Design review of the part built by this model. Coordinates are the model's own, in mm. A direction names the side the tool comes from. Coordinates: 2 decimals unless noted, no trailing zeros. Loops run counter-clockwise (first coordinate to the right, second up) from the corner with the lowest first, then second, coordinate; pieces in that order, holes last. Notation, with made-up numbers: M 18.25,0 L 46.25,0 A31 cw 46.25,26 Z; hole C 63.25,-31 d11. An arc over 180 degrees is marked long. Answer as a JSON object with one key per item and string values. Group by question number.
1. Insertion check: pin 1 (5 mm diameter, centred on x = 16, z = 11, fed in from +Y); pin 2 (2 mm diameter, centred on x = -34.5, z = -5.5, fed in from +Y); pin 3 (1.8 mm diameter, centred on y = 2.5, z = -10.5, fed in from -X); pin 4 (1.9 mm diameter, centred on x = -39.85, z = -29.5, fed in from +Y). Each pin has a flat end and moves straight along its axis. Give the tip position at first contact, or say it passes through.
2. Draft analysis for pull direction X (two halves, no side actions). For faces 1 (the cylindrical face through (29.294, 1.59, -30.383)), 2 (the flat face through (-6, -2, 0)), 3 (the flat face through (12, 4, 22)), 4 (the flat face through (32.54, 2, 0)), state which applies: +X half, -X half, draft (parallel to the pull), parting line (faces both ways), or undercut.
3. Consider section D-D (y = 2.5). State the section outline as (x, z) points.
4. To check wall thickness, follow probe 1 along Z at (x, y) = (14, 2.25); probe 2 along X at (y, z) = (3.25, 0.5); probe 3 along X at (y, z) = (-1, 18). State the ranges of each line that lie inside material, in increasing order.
5. Consider section C-C (x = 20). State the section outline as (y, z) points.
6. Machinability: for faces 5 (the flat face through (-1, 2, 23.04)), 6 (the flat face through (-24.65, -1, 0)), 7 (the flat face through (-6, 5.08, -30)), 8 (the flat face through (-6, 2, -31.748)), 9 (the flat face through (-1, 2, 20.5)), which of the approach directions +Z, -Z, +X, -X, +Y, -Y give a long, thin tool a straight path to every point of the face, cutting with its end or side? Answer none if there is none.
7. Consider section A-A (x = -39.85). State the section outline as (y, z) points.
8. Consider section B-B (z = 17). State the section outline as (x, y) points, then the cut area to 3 significant figures.
Autodesk Inventor part; units mm, degrees
ref_plane "YZ Plane" through (0, 0, 0) normal (1, 0, 0) x (0, 1, 0)
ref_plane "XZ Plane" through (0, 0, 0) normal (0, 1, 0) x (-1, 0, 0)
ref_plane "XY Plane" through (0, 0, 0) normal (0, 0, 1) x (1, 0, 0)
sketch "Sketch1" plane through (0, 0, 0) normal (0, 1, 0) x (-1, 0, 0)
  line L0 (31, 20.5) -> (-30, 20.5)
  line L1 (-30, 20.5) -> (-30, -20.5)
  line L2 (-30, -20.5) -> (31, -20.5)
  line L3 (31, -20.5) -> (31, 20.5)
  line L4 (33.54, 23.04) -> (-32.54, 23.04)
  line L5 (-32.54, 23.04) -> (-32.54, -23.04)
  line L6 (-32.54, -23.04) -> (33.54, -23.04)
  line L7 (33.54, -23.04) -> (33.54, 23.04)
  line L8 (-12, -20.5) -> (-12, 20.5)
  line L9 (-12, -23.04) -> (-12, -20.5)
  line L10 (-12, 20.5) -> (-12, 23.04)
  point P0 (0, 0)
  dimension "d0" = 41
  dimension "d1" = 61
  dimension "d2" = 20.5
  dimension "d3" = 31
  dimension "d4" = 2.54
  dimension "d9" = 18
  dimension "d48" = 46.08
extrude "Extrusion1" add sketch "Sketch1" along normal blind 3.5 contours L0 L10 L4 L7 L6 L9 L2 L3
extrude "Extrusion3" add sketch "Sketch1" along normal blind 5.08 contours L0 L1 L2 L9 L6 L5 L4 L10
sketch "Sketch3" plane through (0, 0, 0) normal (0, -1, 0) x (1, 0, 0)
  line L0 (-31, -20.5) -> (30, -20.5)
  line L1 (-31, 20.5) -> (-31, -20.5)
  line L2 (30, 20.5) -> (-31, 20.5)
  line L3 (30, -20.5) -> (30, 20.5)
  line L4 (32.54, -23.04) -> (-33.54, -23.04)
  line L5 (32.54, 23.04) -> (32.54, -23.04)
  line L6 (-33.54, 23.04) -> (32.54, 23.04)
  line L7 (-33.54, -23.04) -> (-33.54, 23.04)
  point P0 (0, 0)
extrude "Extrusion4" add sketch "Sketch3" along normal blind 1 contours L1 L2 L3 L0 | L4 L7 L6 L5
sketch "Sketch4" plane through (0, 0, 0) normal (0, 1, 0) x (1, 0, 0)
  line L0 (12, -20.5) -> (-31, -20.5)
  line L1 (-31, -20.5) -> (-31, 20.5)
  line L2 (30, 20.5) -> (30, -20.5)
  line L3 (30, -20.5) -> (12, -20.5)
  line L4 (-31, 20.5) -> (12, 20.5)
  line L5 (-24.65, 20.5) -> (-20.459, 20.5)
  line L6 (-20.459, 20.5) -> (-20.459, -20.5)
  line L7 (-20.459, -20.5) -> (-24.65, -20.5)
  line L8 (-24.65, -20.5) -> (-24.65, 20.5)
  line L9 (16.03, -20.5) -> (11.839, -20.5)
  line L10 (11.839, -20.5) -> (11.839, 20.5)
  line L11 (11.839, 20.5) -> (16.03, 20.5)
  line L12 (16.03, 20.5) -> (16.03, -20.5)
  point P0 (0, 0)
  point P1 (-24.65, -20.5)
  dimension "d31" = 4.191
  dimension "d37" = 4.191
  dimension "d38" = 13.97
  dimension "d45" = 6.35
extrude "Extrusion5" cut sketch "Sketch4" against normal blind 25.4 contours L0 L10 L4 L11 L12 L3 | L0 L8 L4 L6
sketch "Sketch6" plane through (0, 0, 0) normal (0, 1, 0) x (1, 0, 0)
  line L0 (30, 20.5) -> (-31, 20.5)
  line L1 (30, -20.5) -> (16.03, -20.5)
  line L2 (30, 20.5) -> (27, 20.5)
  line L3 (27, 20.5) -> (27, -20.5)
  line L4 (27, -20.5) -> (30, -20.5)
  line L5 (30, -20.5) -> (30, 20.5)
  point P0 (0, 0)
  dimension "d33" = 3
extrude "Extrusion7" cut sketch "Sketch6" against normal blind 25.4
sketch "Sketch7" plane through (0, 0, 0) normal (0, 1, 0) x (1, 0, 0)
  line L0 (11.839, -20.5) -> (16.03, -20.5)
  line L1 (27, -20.5) -> (27, 20.5)
  line L2 (16.03, -20.5) -> (27, -20.5)
  line L3 (27, -20.5) -> (27, -16.69)
  line L4 (27, -16.69) -> (16.03, -16.69)
  line L5 (16.03, -16.69) -> (16.03, -20.5)
  line L6 (27, -20.5) -> (16.03, -20.5)
  line L7 (19.6495, -16.69) -> (22.1895, -16.69)
  line L8 (22.1895, -20.5) -> (19.6495, -20.5)
  point P0 (0, 0)
  dimension "d39" = 3.81
  dimension "d41" = 10.97
extrude "Extrusion8" cut sketch "Sketch7" against normal blind 25.4
sketch "Sketch9" plane through (0, -1, 0) normal (0, -1, 0) x (1, 0, 0)
  line L0 (32.54, 31.7522) -> (-43.66, 31.7522)
  line L1 (-43.66, 31.7522) -> (-43.66, -31.7478)
  line L2 (-43.66, -31.7478) -> (32.54, -31.7478)
  line L3 (32.54, -31.7478) -> (32.54, 31.7522)
  line L4 (32.54, -23.04) -> (32.54, 23.04)
  line L5 (-33.54, 23.04) -> (-33.54, -23.04)
  line L6 (27, 16.69) -> (16.03, 16.69)
  line L7 (16.03, 16.69) -> (16.03, -20.5)
  line L8 (16.03, -20.5) -> (11.839, -20.5)
  line L9 (11.839, -20.5) -> (11.839, 20.5)
  line L10 (11.839, 20.5) -> (30, 20.5)
  line L11 (30, 20.5) -> (30, -20.5)
  line L12 (30, -20.5) -> (27, -20.5)
  line L13 (27, -20.5) -> (27, 16.69)
  line L14 (-20.459, 20.5) -> (-20.459, -20.5)
  line L15 (-20.459, -20.5) -> (-24.65, -20.5)
  line L16 (-24.65, -20.5) -> (-24.65, 20.5)
  line L17 (-24.65, 20.5) -> (-20.459, 20.5)
  line L18 (32.54, 23.04) -> (-33.54, 23.04)
  line L19 (-33.54, 23.04) -> (-33.54, -23.04)
  line L20 (-33.54, -23.04) -> (32.54, -23.04)
  line L21 (32.54, -23.04) -> (32.54, 23.04)
  point P0 (0, 0)
  point P1 (-33.54, -23.04)
  dimension "d46" = 0
  dimension "d49" = 8.7122
  dimension "d50" = 63.5
  dimension "d51" = 8.7078
  dimension "d52" = 76.2
extrude "Extrusion9" add sketch "Sketch9" against normal blind 1 contours L3 L18 L5 L20 L2 L1 L0
sketch "Sketch10" plane through (0, 0, 0) normal (0, 1, 0) x (1, 0, 0)
  circle A0 centre (-39.85, 29.4978) radius 1.05
  line L0 (-43.66, 31.7478) -> (-43.66, 27.2478)
  circle A1 centre (-39.85, -29.5022) radius 1.05
  line L1 (-43.66, -27.2522) -> (-43.66, -31.7522)
  circle A2 centre (28.73, 29.4978) radius 1.05
  line L2 (32.54, 27.2478) -> (32.54, 31.7478)
  line L3 (-43.66, 27.2478) -> (32.54, 27.2478)
  circle A3 centre (28.73, -29.5022) radius 1.05
  line L4 (-43.66, -31.7522) -> (32.54, -31.7522)
  line L5 (32.54, -31.7522) -> (32.54, -27.2522)
  line L6 (-43.66, 31.7478) -> (-43.66, -31.7522)
  line L7 (-43.66, -31.7522) -> (32.54, -31.7522)
  line L8 (32.54, 31.7478) -> (32.54, -31.7522)
  line L9 (-43.66, 31.7478) -> (32.54, 31.7478)
  line L10 (-43.66, 31.7478) -> (-43.66, -31.7522)
  line L11 (-43.66, -31.7522) -> (32.54, -31.7522)
  line L12 (32.54, -31.7522) -> (-43.66, -31.7522)
  line L13 (-43.66, -31.7522) -> (-43.66, -27.2522)
  line L14 (-43.66, -27.2522) -> (32.54, -27.2522)
  line L15 (32.54, -27.2522) -> (32.54, -31.7522)
  point P0 (32.54, -0.0022)
  dimension "d55" = 2.1
  dimension "d56" = 3.81
  dimension "d57" = 2.25
  dimension "d58" = 2.25
  dimension "d59" = 2.1
  dimension "d60" = 3.81
  dimension "d61" = 2.1
  dimension "d62" = 2.1
  dimension "d63" = 3.81
  dimension "d64" = 3.81
  dimension "d65" = 2.25
  dimension "d66" = 2.25
  dimension "d67" = 4.5
  dimension "d68" = 4.5
extrude "Extrusion10" add sketch "Sketch10" along normal blind 5.08 contours L9 L2 L3 L0 | L14 L5 L4 L1
sketch "Sketch11" plane through (0, 5.08, 0) normal (0, 1, 0) x (1, 0, 0)
  line L0 (-43.66, 31.7478) -> (-43.66, 27.2478)
  line L1 (-43.66, 27.2478) -> (32.54, 27.2478)
  line L2 (32.54, 27.2478) -> (32.54, 31.7478)
  line L3 (32.54, 31.7478) -> (-43.66, 31.7478)
  circle A0 centre (-39.85, 29.4978) radius 1.05
  circle A1 centre (28.73, 29.4978) radius 1.05
  line L4 (-43.66, -27.2522) -> (-43.66, -31.7522)
  line L5 (-43.66, -31.7522) -> (32.54, -31.7522)
  line L6 (32.54, -31.7522) -> (32.54, -27.2522)
  line L7 (32.54, -27.2522) -> (-43.66, -27.2522)
  circle A2 centre (28.73, -29.5022) radius 1.05
  circle A3 centre (-39.85, -29.5022) radius 1.05
  point P0 (0, 0)
extrude "Extrusion11" cut sketch "Sketch11" against normal blind 25.4 contours A0 | A1 | A2 | A3
sketch "Sketch12" plane through (0, 0, 0) normal (0, 1, 0) x (1, 0, 0)
  line L0 (16.03, -16.69) -> (16.03, 20.5)
  line L1 (27, 20.5) -> (27, -16.69)
  line L2 (16.03, -16.69) -> (27, -16.69)
  line L3 (27, -16.69) -> (27, -14.15)
  line L4 (27, -14.15) -> (16.03, -14.15)
  line L5 (16.03, -14.15) -> (16.03, -16.69)
  line L6 (11.839, 20.5) -> (11.839, -20.5)
  line L7 (11.839, -14.15) -> (16.03, -14.15)
  line L8 (16.03, -14.15) -> (16.03, -6.53)
  line L9 (16.03, -6.53) -> (11.839, -6.53)
  line L10 (11.839, -6.53) -> (11.839, -14.15)
  line L11 (30, -20.5) -> (12, -20.5)
  line L12 (-24.65, -20.5) -> (-24.65, 20.5)
  line L13 (-20.459, -20.5) -> (-20.459, 20.5)
  line L14 (-24.65, -20.5) -> (-20.459, -20.5)
  line L15 (-20.459, -20.5) -> (-20.459, -14.15)
  line L16 (-20.459, -14.15) -> (-24.65, -14.15)
  line L17 (-24.65, -14.15) -> (-24.65, -20.5)
  line L18 (-24.65, 20.5) -> (-20.459, 20.5)
  line L19 (-20.459, 20.5) -> (-20.459, 14.15)
  line L20 (-20.459, 14.15) -> (-24.65, 14.15)
  line L21 (-24.65, 14.15) -> (-24.65, 20.5)
  point P0 (0, 0)
  point P1 (27, -16.69)
  point P2 (11.839, -6.53)
  point P3 (21, -20.5)
  point P4 (13.9345, -14.15)
  dimension "d78" = 2.54
  dimension "d79" = 0
  dimension "d80" = 7.62
  dimension "d81" = 6.35
  dimension "d82" = 6.35
extrude "Extrusion12" cut sketch "Sketch12" against normal blind 25.4 contours L0 L4 L1 L2
extrude "Extrusion13" add sketch "Sketch12" against normal blind 1 contours L7 L6 L9 L0 | L12 L16 L13 L14 | L12 L18 L13 L20
sketch "Sketch13" plane through (0, -1, 0) normal (0, -1, 0) x (1, 0, 0)
  line L0 (11.839, 20.5) -> (-31, 20.5)
  line L1 (16.03, 6.53) -> (16.03, -20.5)
  line L2 (16.03, -20.5) -> (11.839, -20.5)
  line L3 (11.839, -20.5) -> (11.839, 6.53)
  line L4 (11.839, 6.53) -> (16.03, 6.53)
  line L5 (32.54, -31.7478) -> (32.54, 31.7522)
  line L6 (32.54, 31.7522) -> (-43.66, 31.7522)
  line L7 (-43.66, 31.7522) -> (-43.66, -31.7478)
  line L8 (-43.66, -31.7478) -> (32.54, -31.7478)
  line L9 (-20.459, 14.15) -> (-20.459, -14.15)
  line L10 (-20.459, -14.15) -> (-24.65, -14.15)
  line L11 (-24.65, -14.15) -> (-24.65, 14.15)
  line L12 (-24.65, 14.15) -> (-20.459, 14.15)
  line L13 (27, 14.15) -> (11.839, 14.15)
  line L14 (11.839, 14.15) -> (11.839, 20.5)
  line L15 (11.839, 20.5) -> (30, 20.5)
  line L16 (30, 20.5) -> (30, -20.5)
  line L17 (30, -20.5) -> (27, -20.5)
  line L18 (27, -20.5) -> (27, 14.15)
  circle A0 centre (28.73, 29.5022) radius 1.05
  circle A1 centre (28.73, -29.4978) radius 1.05
  circle A2 centre (-39.85, 29.5022) radius 1.05
  circle A3 centre (-39.85, -29.4978) radius 1.05
  point P0 (0, 0)
extrude "Extrusion14" add sketch "Sketch13" along normal blind 1
sketch "Sketch14" plane through (0, 0, 0) normal (0, 1, 0) x (1, 0, 0)
  line L0 (11.839, -14.15) -> (11.839, -20.5)
  line L1 (30, -20.5) -> (30, 20.5)
  line L2 (11.839, -20.5) -> (30, -20.5)
  line L3 (30, -20.5) -> (30, -18.5)
  line L4 (30, -18.5) -> (11.839, -18.5)
  line L5 (11.839, -18.5) -> (11.839, -20.5)
  point P0 (0, 0)
  dimension "d86" = 2
extrude "Extrusion15" add sketch "Sketch14" against normal blind 2
properties part number "RFID_Bottom"
Findings below:
{
 "1": {"pin 1": "stops at y = 0", "pin 2": "stops at y = 3.5", "pin 3": "stops at x = -33.54", "pin 4": "passes through"},
 "2": {"face 1": "undercut", "face 2": "draft", "face 3": "-X half", "face 4": "+X half"},
 "3": {"outline": "M -43.66,-31.75 L 32.54,-31.75 L 32.54,-27.25 L -43.66,-27.25 Z; M -43.66,27.25 L 32.54,27.25 L 32.54,31.75 L -43.66,31.75 Z; M -33.54,-23.04 L 32.54,-23.04 L 32.54,23.04 L -33.54,23.04 Z; hole C -39.85,-29.5 d2.1; hole C -39.85,29.5 d2.1; hole M -31,-20.5 L 30,-20.5 L 30,20.5 L -31,20.5 Z; hole C 28.73,-29.5 d2.1; hole C 28.73,29.5 d2.1"},
 "4": {"probe 1": "z = -31.75 to -27.25, -23.04 to -20.5, 20.5 to 23.04, 27.25 to 31.75", "probe 2": "x = -33.54 to -31, 30 to 32.54", "probe 3": "x = -43.66 to 11.84, 30 to 32.54"},
 "5": {"outline": "M -2,-31.75 L 5.08,-31.75 L 5.08,-27.25 L 0,-27.25 L 0,-23.04 L 5.08,-23.04 L 5.08,-20.5 L 0,-20.5 L 0,14.15 L -2,14.15 Z; M -2,18.5 L 0,18.5 L 0,20.5 L 5.08,20.5 L 5.08,23.04 L 0,23.04 L 0,27.25 L 5.08,27.25 L 5.08,31.75 L -2,31.75 Z"},
 "6": {"face 5": "+X, -X, +Y", "face 6": "+Y, -Y", "face 7": "+Z, -Z, +X, -X, +Y", "face 8": "-Z, +X, -X, +Y, -Y", "face 9": "+Y"},
 "7": {"outline": "M -2,-31.75 L 5.08,-31.75 L 5.08,-30.55 L -2,-30.55 Z; M -2,-28.45 L 5.08,-28.45 L 5.08,-27.25 L 0,-27.25 L 0,27.25 L 5.08,27.25 L 5.08,28.45 L -2,28.45 Z; M -2,30.55 L 5.08,30.55 L 5.08,31.75 L -2,31.75 Z"},
 "8": {"outline": "M -43.66,-2 L 11.84,-2 L 11.84,0 L -31,0 L -31,3.5 L -33.54,3.5 L -33.54,0 L -43.66,0 Z; M 30,-2 L 32.54,-2 L 32.54,5.08 L 30,5.08 Z", "area": "138 mm^2"}
}
